The listing builds one solid part. Answer for the finished solid, in the listing's coordinates (mm). A direction names the side the tool comes from. Give positions to 0.01 mm unless a question says otherwise; leave off trailing zeros. Order: outer loops, then holes, each group sorted by start corner. A loop starts at its lowest first (then second) coordinate and runs counter-clockwise, first axis right, second up. Notation, with made-up numbers: (6, -39.75) - (12, -39.75) arc R14 cw to (12, -20.75) - close; hole circle Ø1 at (-25, 24). An arc over 180 degrees is marked (long way). Write each question's results on one line, items separated by ' | '. Start each with the question number.
1. Section A-A (x = 504) is taken. Give the vertices of the cut face in (y, z), and give its area (3 significant figures).
2. Find the intervals of material crossed by L1, parallel to Z at x = 1929, y = -84; L2, parallel to Z at x = 638, y = -17; L3, parallel to Y at x = 2253.5, z = 2.5, in increasing order.
3. Section C-C (z = -71) is taken. Give the vertices of the cut face in (x, y), and give its area (3 significant figures).
4. Flat-ended cylindrical pins translate along their axes: pin 1 (1 mm diameter, centred on x = 1293, z = -98.5, fed in from -Y); pin 2 (1 mm diameter, centred on x = 239.5, y = -1, fed in from +Z). Find the tip coordinate at first contact, or state that the pin passes through.
5. Section B-B (y = -33.5) is taken. Give the vertices of the cut face in (x, z), and give its area (3 significant figures).
6. Which of the six approach directions +Z, -Z, +X, -X, +Y, -Y give full straight-line access (tool end or side, diameter ignored) to faces 5 (the face through (1380.4, -49.801, -117.706)), 6 (the face through (1380, 0, -2))?
7. Determine the mould class of faces 1 (the face through (1380, -10, 1)), 2 (the face through (2800, -8, 1)), 3 (the face through (1380, -46, -130)), 4 (the face through (1380, -44, 130)) for opening direction Z: released by +Z, released by -Z, zero draft, split by the parting line, or undercut.
from build123d import *

# Parameters (mm, degrees)
EXTRUDE_1_DEPTH     = 2800
SKETCH_3_W          = 3.411754403
SKETCH_3_H          = 3.411754404
CUT_EXTRUDE_1_DEPTH = 0.01
SKETCH_4_W          = 10
SKETCH_4_H          = 10
EXTRUDE_2_DEPTH     = 0.01
SKETCH_4_2_W        = 10
SKETCH_4_2_H        = 10
CUT_EXTRUDE_2_DEPTH = 0.01


with BuildPart() as part:
    # Эскиз2 → Бобышка-Вытянуть1 (new body)
    with BuildSketch(Plane(origin=(0, 0, 0), x_dir=(0, 0, -1), z_dir=(1, 0, 0))):
        with BuildLine():
            Line((130, 0), (-130, 0))
            Line((-130, 0), (-130, -90))
            Line((-130, -90), (-128.678333405, -90))
            ThreePointArc((-128.678333405, -90), (-124.028136062, -88.232175902), (-121.726718983, -83.821618477))
            Line((-121.726718983, -83.821618477), (-113.795983048, -16.720622289))
            ThreePointArc((-113.795983048, -16.720622289), (-108.696165424, -11.795261413), (-101.83727659, -10))
            Line((-101.83727659, -10), (101.83727659, -10))
            ThreePointArc((101.83727659, -10), (108.696165424, -11.795261413), (113.795983048, -16.720622289))
            Line((113.795983048, -16.720622289), (121.726718983, -83.821618477))
            ThreePointArc((121.726718983, -83.821618477), (124.028136062, -88.232175902), (128.678333405, -90))
            Line((128.678333405, -90), (130, -90))
            Line((130, -90), (130, 0))
        make_face()
    extrude(amount=EXTRUDE_1_DEPTH)

    # Эскиз3 → Вырез-Вытянуть1 (cut)
    with BuildSketch(Plane.XY.offset(130)):
        with Locations((239.670222602, -1.705877202)):
            Rectangle(SKETCH_3_W, SKETCH_3_H)
    extrude(amount=-CUT_EXTRUDE_1_DEPTH, mode=Mode.SUBTRACT)

    # Эскиз4 → Бобышка-Вытянуть2 (add)
    with BuildSketch(Plane.XY.offset(130)):
        with Locations((2465, -5)):
            Rectangle(SKETCH_4_W, SKETCH_4_H)
    extrude(amount=-EXTRUDE_2_DEPTH)

    # Эскиз4<2> → Вырез-Вытянуть2 (cut)
    with BuildSketch(Plane.XY.offset(130)):
        with Locations((2465, -5)):
            Rectangle(SKETCH_4_2_W, SKETCH_4_2_H)
    extrude(amount=-CUT_EXTRUDE_2_DEPTH, mode=Mode.SUBTRACT)


solid = part.part
Reported:
1) outline: (-90, -130) - (0, -130) - (0, 130) - (-90, 130) - (-90, 128.68) arc R7 ccw to (-83.82, 121.73) - (-16.72, 113.8) arc R14 cw to (-10, 101.84) - (-10, -101.84) arc R14 cw to (-16.72, -113.8) - (-83.82, -121.73) arc R7 ccw to (-90, -128.68) - close | area: 4,590 mm²
2) L1: -130 to -121.75, 121.75 to 130 | L2: -130 to -113.83, 113.83 to 130 | L3: -10 to 0
3) outline: (0, -10) - (2800, -10) - (2800, 0) - (0, 0) - close | area: 28,000 mm²
4) pin 1: y = -10 | pin 2: z = 129.99
5) outline: (0, -130) - (2800, -130) - (2800, -115.78) - (0, -115.78) - close; (0, 115.78) - (2800, 115.78) - (2800, 130) - (0, 130) - close | area: 79,600 mm²
6) face 5: +X, -X, -Y | face 6: +Z, -Z, +X, -X, +Y
7) face 1: undercut | face 2: zero draft | face 3: released by -Z | face 4: released by +Z
